```python
from build123d import *

# Parameters (mm, degrees)
CROQUIS1_R              = 5
SALIENTE_EXTRUIR1_DEPTH = 220
CROQUIS2_R              = 5
SALIENTE_EXTRUIR2_DEPTH = 10
SALIENTE_EXTRUIR3_START = -10
CROQUIS3_R              = 5
SALIENTE_EXTRUIR3_DEPTH = 10
CROQUIS4_OUTSIDE_W      = 56.09
CROQUIS4_OUTSIDE_H      = 56.09
CROQUIS4_OUTSIDE_R      = 3
CORTAR_EXTRUIR1_DEPTH   = 10
CROQUIS5_OUTSIDE_W      = 56.09
CROQUIS5_OUTSIDE_H      = 56.09
CROQUIS5_OUTSIDE_R      = 3
CORTAR_EXTRUIR2_DEPTH   = 10


with BuildPart() as part:
    # Croquis1 → Saliente-Extruir1 (new body)
    with BuildSketch(Plane(origin=(0, 0, 0), x_dir=(0, 0, -1), z_dir=(1, 0, 0))):
        Circle(CROQUIS1_R)
    extrude(amount=SALIENTE_EXTRUIR1_DEPTH)

    # Croquis2 → Saliente-Extruir2 (add)
    with BuildSketch(Plane.ZY):
        with Locations(Location((0, 0, 0), (0, 0, 180))):
            Circle(CROQUIS2_R)
    extrude(amount=-SALIENTE_EXTRUIR2_DEPTH)

    # Croquis3 → Saliente-Extruir3 (add)
    with BuildSketch(Plane(origin=(220, 0, 0), x_dir=(0, 0, -1), z_dir=(1, 0, 0)).offset(SALIENTE_EXTRUIR3_START)):
        Circle(CROQUIS3_R)
    extrude(amount=SALIENTE_EXTRUIR3_DEPTH)

    # Croquis4 outside → Cortar-Extruir1 (cut)
    with BuildSketch(Plane.ZY):
        Rectangle(CROQUIS4_OUTSIDE_W, CROQUIS4_OUTSIDE_H)
        Circle(CROQUIS4_OUTSIDE_R, mode=Mode.SUBTRACT)
    extrude(amount=-CORTAR_EXTRUIR1_DEPTH, mode=Mode.SUBTRACT)

    # Croquis5 outside → Cortar-Extruir2 (cut)
    with BuildSketch(Plane(origin=(220, 0, 0), x_dir=(0, 0, -1), z_dir=(1, 0, 0))):
        Rectangle(CROQUIS5_OUTSIDE_W, CROQUIS5_OUTSIDE_H)
        with Locations(Location((0, 0, 0), (0, 0, 180))):
            Circle(CROQUIS5_OUTSIDE_R, mode=Mode.SUBTRACT)
    extrude(amount=-CORTAR_EXTRUIR2_DEPTH, mode=Mode.SUBTRACT)


solid = part.part
```
Geometry: final body of the model. Coordinates: model frame, mm. A direction names the side the tool comes from. Give positions to 0.01 mm unless a question says otherwise; leave off trailing zeros. Loops run counter-clockwise (first coordinate to the right, second up) from the corner with the lowest first, then second, coordinate; pieces in that order, holes last. Notation, with made-up numbers: (49.5, 39.25) -> (86.5, 39.25) arc R11 ccw to (86.5, 59.25) -> close; hole circle Ø11 at (30, 89). An arc over 180 degrees is marked (long way). Return JSON: item names as keys, results as strings.
Item 1: Access query for faces 1 (the flat face through (0, 0, 0)), 2 (the flat face through (10, 0.1, 3.3)), 3 (the cylindrical face through (215.07, -0.9, 2.86)). Directions: +Z, -Z, +X, -X, +Y, -Y. A direction counts if a zero-diameter tool reaches every point of the face in a straight line with its end or side. Return the directions, or none.
Filled in:
{"face 1": "+Z, -Z, -X, +Y, -Y", "face 2": "-X", "face 3": "+X"}
Item 2: Section C-C, the plane x = 157.5. Output: boundary loops of the cut face in (y, z).
Filled in:
{"outline": "circle Ø10 at (0, 0)"}
Item 3: Line query: line 1 (X direction, y = 2.5, z = 2.75); line 2 (Y direction, x = 129, z = 4); line 3 (Y direction, x = 159, z = -0.5). Output: solid intervals per line, ascending.
Filled in:
{"line 1": "10 to 210", "line 2": "-3 to 3", "line 3": "-4.97 to 4.97"}
Item 4: Pin query (flat end, axial travel): P1, Ø5, axis at x = 125, z = 2, coming from the -Y side. Return the tip coordinate at first contact, or that it passes through.
Filled in:
{"P1": "y = -5"}
Item 5: Section A-A, the plane z = 0. Output: boundary loops of the cut face in (x, y).
Filled in:
{"outline": "(0, -3) -> (10, -3) -> (10, -5) -> (210, -5) -> (210, -3) -> (220, -3) -> (220, 3) -> (210, 3) -> (210, 5) -> (10, 5) -> (10, 3) -> (0, 3) -> close"}
